Could you check a few things on this model? Use its own coordinates, in mm. A direction names the side the tool comes from. Round coordinates to 2 decimals unless told otherwise and drop trailing zeros. Loops run counter-clockwise (first coordinate to the right, second up) from the corner with the lowest first, then second, coordinate; pieces in that order, holes last. Notation, with made-up numbers: (59, 55.25) -> (80, 55.25) arc R24 cw to (80, 88.25) -> close; hole circle Ø6 at (60, -36). An arc over 180 degrees is marked (long way). Write each question's results on one line, items separated by ' | '.
from build123d import *

# Parameters (mm, degrees)
F0_R     = 7.002159
F1_DEPTH = 25.4


with BuildPart() as f1:
    # F0 (on Front) → F1 (new body)
    with BuildSketch(Plane.XZ):
        with BuildLine():
            ThreePointArc((4.748446, 26.716104), (9.565493, 30.908048), (11.360195, 37.036292))
            ThreePointArc((11.360195, 37.036292), (-6.561535, 46.309926), (-3.78044, 26.323575))
            ThreePointArc((-3.78044, 26.323575), (0.522282, 25.688109), (4.748446, 26.716104))
        make_face()
        with Locations((0, 37.036292)):
            Circle(F0_R, mode=Mode.SUBTRACT)
        with BuildLine():
            ThreePointArc((4.748446, 26.716104), (0.522282, 25.688109), (-3.78044, 26.323575))
            Line((-3.78044, 26.323575), (-3.78044, 0))
            Line((-3.78044, 0), (-3.78044, -3.634142))
            Line((-3.78044, -3.634142), (-3.78044, -13.665396))
            Line((-3.78044, -13.665396), (-3.78044, -16.9164))
            Line((-3.78044, -16.9164), (-3.78044, -20.276576))
            Line((-3.78044, -20.276576), (4.748446, -20.276576))
            Line((4.748446, -20.276576), (4.748446, 26.716104))
        make_face()
        Polygon((-3.78044, -3.634142), (-3.78044, 0), (-15.900498, 0), (-15.900498, -6.099688), (-10.969408, -6.099688), (-10.969408, -3.634142), align=None)
        Polygon((-3.78044, -16.9164), (-3.78044, -13.665396), (-10.969408, -13.665396), (-10.969408, -10.414393), (-15.900498, -10.414393), (-15.900498, -16.9164), align=None)
    extrude(amount=F1_DEPTH)


solid = f1.part
1) I'm going to push flat-ended pins straight in: pin 1 (7.5 mm diameter, centred on y = -15, z = 10.5, fed in from -X); pin 2 (8 mm diameter, centred on y = -10, z = 24, fed in from +X); pin 3 (5.5 mm diameter, centred on x = -12.5, y = -9, fed in from -Z). Where does each tip first touch, or does it pass through?
Model answer:
pin 1: stops at x = -3.78 | pin 2: stops at x = 6.88 | pin 3: stops at z = -16.92
2) I want a section at D-D, the plane x = -4.75. Write out the boundary of the cut face in (y, z), plus the area to 3 significant figures.
Model answer:
outline: (-25.4, -16.92) -> (0, -16.92) -> (0, -13.67) -> (-25.4, -13.67) -> close; (-25.4, -3.63) -> (0, -3.63) -> (0, 0) -> (-25.4, 0) -> close; (-25.4, 26.72) -> (0, 26.72) -> (0, 31.89) -> (-25.4, 31.89) -> close; (-25.4, 42.18) -> (0, 42.18) -> (0, 47.36) -> (-25.4, 47.36) -> close | area: 438 mm2
3) I want a section at B-B, the plane y = -12. Write out the boundary of the cut face in (x, z).
Model answer:
outline: (-15.9, -16.92) -> (-3.78, -16.92) -> (-3.78, -20.28) -> (4.75, -20.28) -> (4.75, 26.72) arc R11.36 ccw to (11.36, 37.04) arc R11.36 ccw (long way) to (-3.78, 26.32) -> (-3.78, 0) -> (-15.9, 0) -> (-15.9, -6.1) -> (-10.97, -6.1) -> (-10.97, -3.63) -> (-3.78, -3.63) -> (-3.78, -13.67) -> (-10.97, -13.67) -> (-10.97, -10.41) -> (-15.9, -10.41) -> close; hole circle Ø14 at (0, 37.04)
4) I need wall thicknesses on line 1 (Z direction, x = 0, y = -17.75); line 2 (X direction, y = -6.75, z = -12); line 3 (Z direction, x = -14.25, y = -2). Which ranges of each line are inside material? Lowest first, please.
Model answer:
line 1: z = -20.28 to 30.03, 44.04 to 48.4 | line 2: x = -15.9 to -10.97, -3.78 to 4.75 | line 3: z = -16.92 to -10.41, -6.1 to 0
5) I want a section at A-A, the plane z = -13. Write out the boundary of the cut face in (x, y), plus the area to 3 significant figures.
Model answer:
outline: (-15.9, -25.4) -> (-10.97, -25.4) -> (-10.97, 0) -> (-15.9, 0) -> close; (-3.78, -25.4) -> (4.75, -25.4) -> (4.75, 0) -> (-3.78, 0) -> close | area: 342 mm2
6) I want a section at C-C, the plane x = 0. Write out the boundary of the cut face in (y, z), plus the area to 3 significant figures.
Model answer:
outline: (-25.4, -20.28) -> (0, -20.28) -> (0, 30.03) -> (-25.4, 30.03) -> close; (-25.4, 44.04) -> (0, 44.04) -> (0, 48.4) -> (-25.4, 48.4) -> close | area: 1,390 mm2
7) If we mould it in two halves opening along Z, with no side actions, what happens to faces 1 (the flat face through (4.748, -13, 3)), 2 (the flat face through (-7, -13, -3.634)), 3 (the flat face through (-7, -13, -13.665)), 4 (the flat face through (0, -13, -20.277))? For each: released by +Z, released by -Z, zero draft, split by the parting line, or undercut.
Model answer:
face 1: zero draft | face 2: undercut | face 3: undercut | face 4: released by -Z
8) For faces 5 (the flat face through (-10.969, -13, -12)), 6 (the flat face through (-3.78, -13, -19)), 7 (the flat face through (-3.78, -13, 13)), which set-ups out of +Z, -Z, +X, -X, +Y, -Y let a thin tool reach every point of the face, with its end or its side?
Model answer:
face 5: +Y, -Y | face 6: -Z, -X, +Y, -Y | face 7: -X, +Y, -Y
